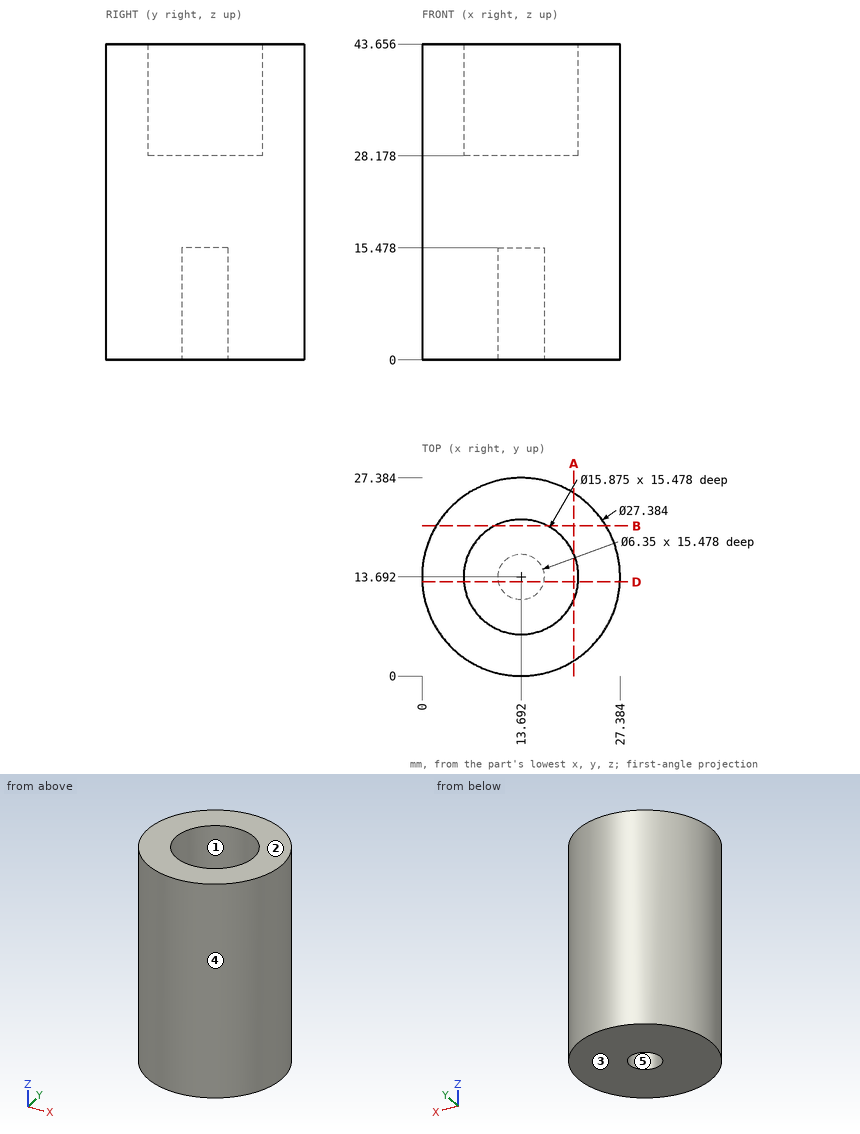
Verification items for this drawing (mm, ordinates from the low corner). A direction names the side the tool comes from. Coordinates: 2 decimals unless noted, no trailing zeros. Loops run counter-clockwise (first coordinate to the right, second up) from the corner with the lowest first, then second, coordinate; pieces in that order, holes last. Notation, with made-up numbers: (-22, 30.25) - (-13, 30.25) arc R22 cw to (-13, 36.25) - close; hole circle Ø5 at (1.25, 87). An arc over 180 degrees is marked (long way). One line per item, written item: value. Start each with the question number.
(1) Depth check by flat-ended pin: P1, Ø5, axis at x = 13.69, y = 13.69, coming from the +Z side; P2, Ø3, axis at y = 4.5, z = 32.5, coming from the +X side; P3, Ø1, axis at x = 16, y = 14, coming from the -Z side. Enter the tip coordinate at first touch or a pass-through.
(2) Mould release check, pull along X, two halves, no side actions. Record for the marked faces 3, 4 and 5: released by +X, released by -X, zero draft, split by the parting line, or undercut.
(3) Cross-section at A-A on x = 21. Enter the section's corners in (y, z).
(4) Cross-section at B-B on y = 20.75. Enter the section's corners in (x, z) (1 decimal), plus the area to 3 significant figures.
(5) Material ranges on line 1 (Y direction, x = 16, z = 41.5) (1 decimal); line 2 (Z direction, x = 19.5, y = 14.5); line 3 (X direction, y = 12.75, z = 30.5), recorded low to high. Write a range as [from, to].
(6) Tool access check on the marked faces 1 and 2. Record the directions out of +Z, -Z, +X, -X, +Y, -Y that give a thin tool (end or side, any length) a straight path to the whole face; none if there is none.
(7) Cross-section at D-D on y = 13. Enter the section's corners in (x, z) (1 decimal), plus the area to 3 significant figures.
Results below:
1. P1: stops at z = 28.18
1. P2: stops at x = 25.02
1. P3: stops at z = 15.48
2. face 3: zero draft
2. face 4: split by the parting line
2. face 5: undercut
3. outline: (2.11, 0) - (25.27, 0) - (25.27, 43.66) - (16.79, 43.66) - (16.79, 28.18) - (10.59, 28.18) - (10.59, 43.66) - (2.11, 43.66) - close
4. outline: (2, 0) - (25.4, 0) - (25.4, 43.7) - (17.3, 43.7) - (17.3, 28.2) - (10.1, 28.2) - (10.1, 43.7) - (2, 43.7) - close
4. area: 912 mm2
5. line 1: y = [0.2, 6.1], [21.3, 27.2]
5. line 2: z = [0, 28.18]
5. line 3: x = [0.03, 5.81], [21.57, 27.35]
6. face 1: +Z
6. face 2: +Z, +X, -X, +Y, -Y
7. outline: (0, 0) - (10.6, 0) - (10.6, 15.5) - (16.8, 15.5) - (16.8, 0) - (27.4, 0) - (27.4, 43.7) - (21.6, 43.7) - (21.6, 28.2) - (5.8, 28.2) - (5.8, 43.7) - (0, 43.7) - close
7. area: 853 mm2
